from build123d import *

# Parameters (mm, degrees)
SKETCH1_R             = 1.25
BOSS_EXTRUDE1_DEPTH   = 7.9
CUT_EXTRUDE2_DEPTH    = 61.929549481
M3X0_5_TAPPED_HOLE1_D = 2.5
SKETCH7_W             = 8
SKETCH7_H             = 0.5
CUT_EXTRUDE3_DEPTH    = 61.929549481
SKETCH8_R             = 2
CUT_EXTRUDE4_DEPTH    = 57.217523958
CUT_EXTRUDE5_DEPTH    = 3
CUT_EXTRUDE6_DEPTH    = 1
CUT_EXTRUDE8_DEPTH    = 3.9


with BuildPart() as part:
    # Sketch1 → Boss-Extrude1 (new body)
    with BuildSketch(Plane(origin=(0, 0, 0), x_dir=(0, 0, -1), z_dir=(1, 0, 0))):
        with BuildLine():
            Line((0, 0), (0, 16))
            Line((0, 16), (-23.49505807, 51.650837947))
            ThreePointArc((-23.49505807, 51.650837947), (-27.398738146, 52.653965259), (-28.777698581, 48.866690426))
            Line((-28.777698581, 48.866690426), (-17, 20))
            Line((-17, 20), (-17, 0))
            Line((-17, 0), (0, 0))
        make_face()
        with Locations((-26, 50)):
            Circle(SKETCH1_R, mode=Mode.SUBTRACT)
    extrude(amount=BOSS_EXTRUDE1_DEPTH)

    # Sketch3 → Cut-Extrude2 (cut, through all)
    with BuildSketch(Plane(origin=(0, 0, 0), x_dir=(-1, 0, 0), z_dir=(0, 0, -1))):
        Polygon((-7.9, 0), (-4.9, 0), (-2.9, 4), (-7.9, 4), align=None)
    extrude(amount=-CUT_EXTRUDE2_DEPTH, mode=Mode.SUBTRACT)

    # M3x0.5 Tapped Hole1 (through all)
    with Locations(Plane(origin=(7.9, 7, 3), x_dir=(0, 0, 1), z_dir=(1, 0, 0))):
        with Locations((0, 0)):
            Hole(M3X0_5_TAPPED_HOLE1_D / 2)

    # Sketch7 → Cut-Extrude3 (cut, through all)
    with BuildSketch(Plane(origin=(0, 0, 0), x_dir=(-1, 0, 0), z_dir=(0, 0, -1))):
        with Locations((-4, 0.25)):
            Rectangle(SKETCH7_W, SKETCH7_H)
    extrude(amount=-CUT_EXTRUDE3_DEPTH, mode=Mode.SUBTRACT)

    # Sketch8 → Cut-Extrude4 (cut, through all)
    with BuildSketch(Plane.XY.offset(17)):
        with Locations((3.9, 12)):
            Circle(SKETCH8_R)
    extrude(amount=-CUT_EXTRUDE4_DEPTH, mode=Mode.SUBTRACT)

    # Sketch9 → Cut-Extrude5 (cut)
    with BuildSketch(Plane(origin=(0, 0, 0), x_dir=(-1, 0, 0), z_dir=(0, 0, -1))):
        Polygon((-4.65, 0.5), (-2.9, 4), (0, 4), (0, 0.5), align=None)
    extrude(amount=-CUT_EXTRUDE5_DEPTH, mode=Mode.SUBTRACT)

    # Sketch11 → Cut-Extrude6 (cut)
    with BuildSketch(Plane.ZY):
        with BuildLine():
            Line((0, 16), (17, 20))
            Line((17, 20), (28.777698581, 48.866690426))
            ThreePointArc((28.777698581, 48.866690426), (27.398738146, 52.653965259), (23.49505807, 51.650837947))
            Line((23.49505807, 51.650837947), (0, 16))
        make_face()
    extrude(amount=-CUT_EXTRUDE6_DEPTH, mode=Mode.SUBTRACT)

    # Sketch14 → Cut-Extrude8 (cut, symmetric)
    with BuildSketch(Plane.ZY.offset(-1)):
        with BuildLine():
            Line((0, 16), (15.958100151, 40.214438659))
            ThreePointArc((15.958100151, 40.214438659), (15.69103598, 23.024770582), (0, 16))
        make_face()
    extrude(amount=CUT_EXTRUDE8_DEPTH, both=True, mode=Mode.SUBTRACT)


solid = part.part
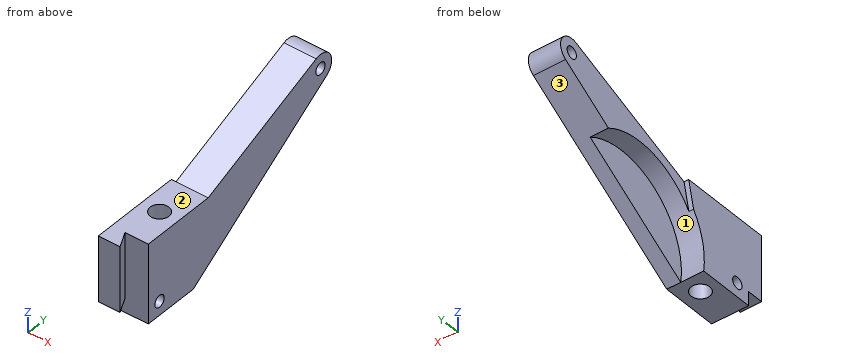
Design review of the part built by this model. Coordinates are the model's own, in mm. Face numbers are marked on the shaded views. A direction names the side the tool comes from. Round coordinates to 2 decimals unless told otherwise and drop trailing zeros. Order: outer loops, then holes, each group sorted by start corner. A loop starts at its lowest first (then second) coordinate and runs counter-clockwise, first axis right, second up. Notation, with made-up numbers: M 83,40 L 114,40 A20 cw 114,68 Z; hole C -36.75,10 d2. An arc over 180 degrees is marked long. Answer as CSV lines item,"result". Start each with the question number.
1) Add section B-B (x = 3.9). Give the boundary of the cut face in (y, z), then the cut area to 3 significant figures.
2) Wall thickness on line 1 along Y through (x, z) = (2.75, 16.5); line 2 along Y through (x, z) = (3.9, 3.75); line 3 along Y through (x, z) = (5, 15.75): over which ranges is each line inside the solid? List them lowest first. Write a range as [from, to].
3) Add section A-A (y = 7). Give the boundary of the cut face in (x, z), then the cut area to 3 significant figures.
4) For pin 1 Ø14 at (y, z) = (40, 21) entering from -X; pin 2 Ø3 at (x, y) = (3.5, 44) entering from -Z; pin 3 Ø2 at (y, z) = (35, 13.5) entering from -X; pin 4 Ø1 at (y, z) = (11, 9.5) entering from -X, all flat-tipped, find the tip position at first contact; note any pin that passes through.
5) Add section C-C (z = 14.5). Give the boundary of the cut face in (x, y), then the cut area to 3 significant figures.
6) Add section D-D (x = 0.5). Give the boundary of the cut face in (y, z).
7) Tool access review of the marked faces 1, 2 and 3: name each direction out of +Z, -Z, +X, -X, +Y, -Y from which nothing blocks a thin tool from reaching the whole face with its end or side.
Resolved:
1,outline,"M 0.5,3 L 2,3 L 2,17 L 0.5,17 Z; M 4,0 L 10,0 L 10,17 L 4,17 Z; M 14,0 L 16,0 A16 cw 40.21,15.96 L 51.65,23.5 A3 ccw 48.87,28.78 L 20,17 L 14,17 Z; hole C 7,3 d2.5; hole C 50,26 d2.5"
1,area,"350 mm^2"
2,line 1,"[0.5, 10.36], [13.64, 24.4], [39.26, 41.04]"
2,line 2,"[0.5, 2], [4, 6], [8, 10], [14, 15.89]"
2,line 3,"[4, 10.33], [13.67, 39.9]"
3,outline,"M 0,0 L 7.9,0 L 7.9,1.75 L 0,1.75 Z; M 0,4.25 L 7.9,4.25 L 7.9,17 L 0,17 Z"
3,area,"115 mm^2"
4,pin 1,"x = 1"
4,pin 2,"z = 17.46"
4,pin 3,"x = 4.9"
4,pin 4,"x = 0"
5,outline,"M 0,0.5 L 4.65,0.5 L 2.9,4 L 7.9,4 L 7.9,38 L 4.9,38 L 4.9,21.44 L 1,21.44 L 1,19.41 L 0,19.41 Z; hole C 3.9,12 d4"
5,area,"186 mm^2"
6,outline,"M 0.5,3 L 4,3 L 4,0 L 16,0 A16 cw 18.7,11.48 L 20,17 L 0.5,17 Z; hole C 7,3 d2.5"
7,face 1,"-X"
7,face 2,"+Z, +X, -X, -Y"
7,face 3,"-Z, +X, -X, +Y"
